Design review of the part built by this model. Coordinates are the model's own, in mm. Face numbers are marked on the shaded views. A direction names the side the tool comes from. Give positions to 0.01 mm unless a question says otherwise; leave off trailing zeros. Write each loop counter-clockwise with the first axis right and the second up, starting at its lowest first coordinate (ties: lowest second). Pieces come first, ordered by that corner, then holes. Notation, with made-up numbers: (20.25, -4) -> (71.25, -4) arc R5 ccw to (71.25, 3) -> close; hole circle Ø8 at (84.25, 10). An arc over 180 degrees is marked (long way). Return JSON: item names as keys, results as strings. Group by question number.
from build123d import *

# Parameters (mm, degrees)
F2_W          = 5.7
F2_H          = 2.4
F3_DEPTH      = 6.5
F4_R          = 1.75
F5_DEPTH      = 10.743375338
F5_DEPTH_BACK = 3.658624662
F6_R          = 0.5


with BuildPart() as f1:
    # F0 (on Front) → F1 (revolve)
    with BuildSketch(Plane.XZ):
        Polygon((-7.2, 0), (-3.1, 0), (-3.1, 15.5), (-7.2, 15.5), (-7.2, 8.5), (-6.2, 8.5), (-6.2, 1), (-7.2, 1), align=None)
    revolve(axis=Axis((0, 0, 7.75), (0, 0, -1)))

    # F2 (on face) → F3 (cut)
    with BuildSketch(Plane.XY.offset(15.5)):
        with Locations((0, -4.742375338)):
            Rectangle(F2_W, F2_H)
        with Locations((0, 4.742375338)):
            Rectangle(F2_W, F2_H)
    extrude(amount=-F3_DEPTH, mode=Mode.SUBTRACT)

    # F4 (on face) → F5 (cut, two sides)
    with BuildSketch(Plane.XZ.offset(3.542375338)) as f5_sk:
        with Locations((0, 12.25)):
            Circle(F4_R)
    extrude(amount=-F5_DEPTH, mode=Mode.SUBTRACT)
    extrude(f5_sk.sketch, amount=F5_DEPTH_BACK, mode=Mode.SUBTRACT)

    # F6
    f6_edges = [f1.edges().sort_by_distance(p)[0] for p in [
        (7.2, 0, 0),
        (7.2, 0, 15.5),
        (3.1, 0, 0),
    ]]
    fillet(f6_edges, radius=F6_R)


solid = f1.part
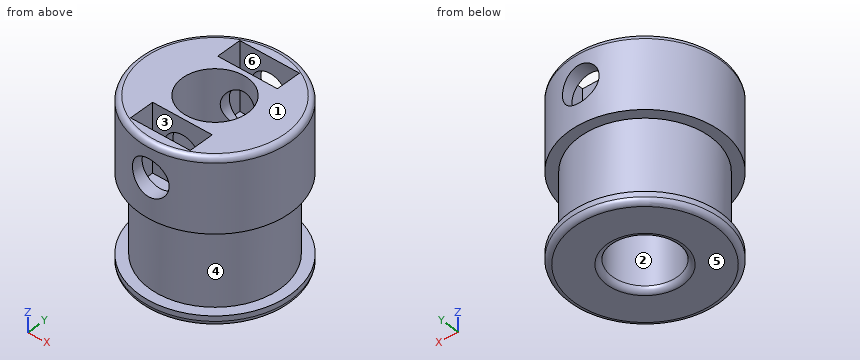
Q1. Take a section at A-A, the plane y = 0. Give the boundary of the cut face in (x, z), plus the area to 3 significant figures.
Q2. Tool access review of the marked faces 5 and 6: name each direction out of +Z, -Z, +X, -X, +Y, -Y from which nothing blocks a thin tool from reaching the whole face with its end or side.
Q3. Take a section at C-C, the plane x = 0. Count the separate pieces of the cut face and the enclosed holes in it, plus the area to 3 significant figures.
Q4. Take a section at B-B, the plane z = 11.75. Give the boundary of the cut face in (x, y), plus the area to 3 significant figures.
Q5. Mouldability with a two-part tool opening along Y and no side actions: class the marked faces 1, 2, 3 and 4 as +Y half, -Y half, draft (parallel to the pull), parting line (faces both ways), or undercut.
Q6. For L1, parallel to Z at x = 0, y = -6.7; L2, parallel to Y at x = 0, z = 9.5; L3, parallel to Y at x = -1.25, z = 15, list the stretches that pass through material, from the lowest coordinate up. Write a range as from..to.
Q7. Insertion check: pin 1 (0.7 mm diameter, centred on y = -5, z = 13.5, fed in from +X); pin 2 (2.5 mm diameter, centred on y = 4, z = 12, fed in from -X); pin 3 (3 mm diameter, centred on x = -3, y = 0, fed in from -Z); pin 4 (0.7 mm diameter, centred on x = -1, y = -4.5, fed in from +Z). Each pin has a flat end and moves straight along its axis. Give the tip position at first contact, or say it passes through.
Final values:
{
 "1": {"outline": "(-7.2, 0.5) arc R0.5 ccw to (-6.7, 0) -> (-3.6, 0) arc R0.5 ccw to (-3.1, 0.5) -> (-3.1, 15.5) -> (-6.7, 15.5) arc R0.5 ccw to (-7.2, 15) -> (-7.2, 8.5) -> (-6.2, 8.5) -> (-6.2, 1) -> (-7.2, 1) -> close; (3.1, 0.5) arc R0.5 ccw to (3.6, 0) -> (6.7, 0) arc R0.5 ccw to (7.2, 0.5) -> (7.2, 1) -> (6.2, 1) -> (6.2, 8.5) -> (7.2, 8.5) -> (7.2, 15) arc R0.5 ccw to (6.7, 15.5) -> (3.1, 15.5) -> close", "area": "112 mm²"},
 "2": {"face 5": "-Z, +X, -X, +Y, -Y", "face 6": "+Z"},
 "3": {"separate pieces": "6", "enclosed holes": "0", "area": "68.7 mm²"},
 "4": {"outline": "(-2.85, -5.94) -> (-2.85, -3.54) -> (-1.68, -3.54) -> (-1.68, -2.61) arc R3.1 cw to (-1.68, 2.61) -> (-1.68, 3.54) -> (-2.85, 3.54) -> (-2.85, 5.94) -> (-1.68, 5.94) -> (-1.68, 7) arc R7.2 ccw to (-1.68, -7) -> (-1.68, -5.94) -> close; (1.68, -7) arc R7.2 ccw to (1.68, 7) -> (1.68, 5.94) -> (2.85, 5.94) -> (2.85, 3.54) -> (1.68, 3.54) -> (1.68, 2.61) arc R3.1 cw to (1.68, -2.61) -> (1.68, -3.54) -> (2.85, -3.54) -> (2.85, -5.94) -> (1.68, -5.94) -> close", "area": "93.3 mm²"},
 "5": {"face 1": "draft", "face 2": "undercut", "face 3": "undercut", "face 4": "parting line"},
 "6": {"L1": "z = 0..1, 8.5..10.5, 14..15.5", "L2": "y = -7.2..-5.94, -3.54..-3.1, 3.1..3.54, 5.94..7.2", "L3": "y = -7.09..-5.94, -3.54..-2.84, 2.84..3.54, 5.94..7.09"},
 "7": {"pin 1": "stops at x = 5.5", "pin 2": "stops at x = -6.65", "pin 3": "stops at z = 0", "pin 4": "stops at z = 9"}
}
